Input: part model. Units: mm. Frame: model coordinates. A direction names the side the tool comes from. Coordinates: 2 decimals unless noted, no trailing zeros. Loops run counter-clockwise (first coordinate to the right, second up) from the corner with the lowest first, then second, coordinate; pieces in that order, holes last.
(1) Section C-C, the plane y = 2.65. Return loops of the section in (x, z).
(2) Set-up query: faces 5 (the face through (-8, 0, -12)), 6 (the face through (35, 2, 23)). Return all of +Z, -Z, +X, -X, +Y, -Y with unobstructed straight access to the full face (end or side cutting, diameter ignored); none if empty.
(3) Section A-A, the plane x = 17. Return loops of the section in (y, z), then the cut area to 3 significant figures.
(4) Section B-B, the plane z = 8. Return loops of the section in (x, y).
(5) Line query: L1, parallel to X at y = 2.3, z = 38; L2, parallel to Z at x = 18, y = 2.25. Output: solid intervals per line, ascending.
(6) Mould query, pull axis Z, two halves, no side actions, for faces 1 (the face through (10, 2, 58.5)), 2 (the face through (37.5, 2, 2)), 3 (the face through (-15.1, 2, 24)), 4 (the face through (-1, 2, 61)). Classes: released by +Z, released by -Z, zero draft, split by the parting line, or undercut.
Autodesk Inventor part; units mm, degrees
ref_plane "YZ Plane" through (0, 0, 0) normal (1, 0, 0) x (0, 1, 0)
ref_plane "XZ Plane" through (0, 0, 0) normal (0, 1, 0) x (-1, 0, 0)
ref_plane "XY Plane" through (0, 0, 0) normal (0, 0, 1) x (1, 0, 0)
sketch "Sketch2" plane through (0, 0, 0) normal (0, 1, 0) x (-1, 0, 0)
  line L0 (37.5, 59.5) -> (-37.5, 59.5)
  line L1 (-37.5, 59.5) -> (-37.5, -59.5)
  line L2 (-37.5, -59.5) -> (37.5, -59.5)
  line L3 (37.5, -59.5) -> (37.5, 59.5)
  line L4 (37.5, 59.5) -> (-37.5, -59.5) construction
  line L5 (-37.5, 59.5) -> (37.5, -59.5) construction
  line L6 (-35, 58.5) -> (15.1, 58.5)
  line L7 (15.1, 58.5) -> (15.1, -11.6)
  line L8 (15.1, -11.6) -> (-35, -11.6)
  line L9 (-35, -11.6) -> (-35, 58.5)
  line L10 (-37.5, 59.5) -> (37.5, 59.5)
  line L11 (37.5, 59.5) -> (37.5, 61)
  line L12 (37.5, 61) -> (-37.5, 61)
  line L13 (-37.5, 61) -> (-37.5, 59.5)
  point P0 (0, 0)
  dimension "d8" = 119
  dimension "d9" = 75
  dimension "d10" = 2.5
  dimension "d11" = 1
  dimension "d12" = 70.1
  dimension "d13" = 50.1
  dimension "d14" = 1.5
extrude "Extrusion2" add sketch "Sketch2" along normal blind 3.9
properties part number "lid" material "Acetal Resin, Black"
Report:
1. outline: (-37.5, -59.5) - (37.5, -59.5) - (37.5, 61) - (-37.5, 61) - close; hole (-15.1, -11.6) - (35, -11.6) - (35, 58.5) - (-15.1, 58.5) - close
2. face 5: +Z, -Z, +X, -X, -Y
2. face 6: +Y, -Y
3. outline: (0, -59.5) - (3.9, -59.5) - (3.9, -11.6) - (0, -11.6) - close; (0, 58.5) - (3.9, 58.5) - (3.9, 61) - (0, 61) - close
3. area: 197 mm2
4. outline: (-37.5, 0) - (-15.1, 0) - (-15.1, 3.9) - (-37.5, 3.9) - close; (35, 0) - (37.5, 0) - (37.5, 3.9) - (35, 3.9) - close
5. L1: x = -37.5 to -15.1, 35 to 37.5
5. L2: z = -59.5 to -11.6, 58.5 to 61
6. face 1: undercut
6. face 2: zero draft
6. face 3: undercut
6. face 4: released by +Z
